Build history of the part. All positions in model axes, mm. Face numbers are marked on the shaded views. A direction names the side the tool comes from. Round coordinates to 2 decimals unless told otherwise and drop trailing zeros. Write each loop counter-clockwise with the first axis right and the second up, starting at its lowest first coordinate (ties: lowest second). Pieces come first, ordered by that corner, then holes.
Item 1: Wall check: probe 1 along Y at (x, z) = (11, 4); probe 2 along Y at (x, z) = (18, 10); probe 3 along Z at (x, y) = (1.5, -13). Give the ranges that are in metal, low to high.
Item 2: 3-axis set-ups, long thin cutter, end or side, ignore diameter. For the marked faces 4, 5, 6 and 7: which of +Z, -Z, +X, -X, +Y, -Y reach the whole face in a straight line?
Item 3: Band-saw the part on B-B, the plane x = 21.5. Write the cut outline in (y, z), then the cut area to 3 significant figures.
Item 4: Band-saw the part on A-A, the plane y = 25. Write the cut outline in (x, z).
Item 5: Drop flat-ended pins along their axis: pin 1 Ø3 at (x, y) = (17, -3) entering from -Z; pin 2 Ø5 at (y, z) = (-24, 3) entering from +X; pin 3 Ø2 at (x, z) = (21, 9.5) entering from +Y. Give the stop position or say it passes through.
Item 6: Band-saw the part on D-D, the plane x = -7.2. Count the separate pieces of the cut face and the enclosed holes in it, then the cut area to 3 significant figures.
Item 7: Mould opens along Z. For the marked faces 1, 2 and 3 say: +Z half, -Z half, draft (parallel to the pull), parting line (faces both ways), or undercut.
Item 8: Band-saw the part on C-C, the plane z = 10. Write the cut outline in (x, y), then the cut area to 3 significant figures.
```python
from build123d import *

# Parameters (mm, degrees)
CROQUIS1_W             = 99.2
CROQUIS1_H             = 47
BASE_DEPTH             = 17.6
CROQUIS2_W             = 30.4
CROQUIS2_H             = 14.4
PLATES_DEPTH           = 40.8
CROQUIS4_W             = 2
CROQUIS4_H             = 2.8
WINDOW_LATERAL_1_DEPTH = 40.8
CROQUIS5_R             = 2
WINDOW_LATERAL_2_DEPTH = 2
WINDOW_LATERAL_3_START = -2
WINDOW_LATERAL_3_DEPTH = 2
CROQUIS7_W             = 30.4
CROQUIS7_H             = 2.8
WINDOW_BEHIND_1_DEPTH  = 6.2
WINDOW_BEHIND_2_DEPTH  = 59.973892529
CROQUIS9_R             = 2
WINDOW_BEHIND_3_DEPTH  = 59.973892529
WINDOW_BOTTOM_DEPTH    = 59.973892529
ROTOR_JOIN_1_DEPTH     = 4
CROQUIS12_R            = 1.4
ROTOR_JOIN_2_DEPTH     = 10.2
ROTOR_LIMIT_1_DEPTH    = 16
ROTOR_LIMIT_2_DEPTH    = 16


with BuildPart() as part:
    # Croquis1 → BASE (new body)
    with BuildSketch(Plane(origin=(0, 0, 0), x_dir=(0, 1, 0), z_dir=(0, 0, 1))):
        with Locations((0, 4.1)):
            Rectangle(CROQUIS1_W, CROQUIS1_H)
    extrude(amount=BASE_DEPTH)

    # Croquis2 → PLATES (cut)
    with BuildSketch(Plane(origin=(-27.6, 0, 0), x_dir=(0, -1, 0), z_dir=(-1, 0, 0))):
        with Locations((-32.4, 8.8)):
            Rectangle(CROQUIS2_W, CROQUIS2_H)
        with Locations((0, 8.8)):
            Rectangle(CROQUIS2_W, CROQUIS2_H)
        with Locations((32.4, 8.8)):
            Rectangle(CROQUIS2_W, CROQUIS2_H)
    extrude(amount=-PLATES_DEPTH, mode=Mode.SUBTRACT)

    # Croquis4 → WINDOW_LATERAL_1 (cut)
    with BuildSketch(Plane(origin=(-27.6, 0, 0), x_dir=(0, -1, 0), z_dir=(-1, 0, 0))):
        with Locations((48.6, 14.6)):
            Rectangle(CROQUIS4_W, CROQUIS4_H)
        with Locations((-48.6, 14.6)):
            Rectangle(CROQUIS4_W, CROQUIS4_H)
    extrude(amount=-WINDOW_LATERAL_1_DEPTH, mode=Mode.SUBTRACT)

    # Croquis5 → WINDOW_LATERAL_2 (cut)
    with BuildSketch(Plane.XZ.offset(49.6)):
        with Locations((-7.2, 13.2)):
            Circle(CROQUIS5_R)
    extrude(amount=-WINDOW_LATERAL_2_DEPTH, mode=Mode.SUBTRACT)

    # Croquis6 → WINDOW_LATERAL_3 (cut)
    with BuildSketch(Plane(origin=(0, 49.6, 0), x_dir=(-1, 0, 0), z_dir=(0, 1, 0)).offset(WINDOW_LATERAL_3_START)):
        with BuildLine():
            Line((9.2, 13.2), (5.2, 13.2))
            ThreePointArc((5.2, 13.2), (7.2, 11.2), (9.2, 13.2))
        make_face()
    extrude(amount=WINDOW_LATERAL_3_DEPTH, mode=Mode.SUBTRACT)

    # Croquis7 → WINDOW_BEHIND_1 (cut)
    with BuildSketch(Plane(origin=(13.2, 0, 0), x_dir=(0, -1, 0), z_dir=(-1, 0, 0))):
        with Locations((0, 3)):
            Rectangle(CROQUIS7_W, CROQUIS7_H)
    extrude(amount=-WINDOW_BEHIND_1_DEPTH, mode=Mode.SUBTRACT)

    # Croquis8 → WINDOW_BEHIND_2 (cut, through all)
    with BuildSketch(Plane.XY.offset(1.6)):
        with BuildLine():
            Line((15.2, -11), (15.2, 11))
            ThreePointArc((15.2, 11), (19.4, 15.2), (23.6, 11))
            Line((23.6, 11), (23.6, -11))
            ThreePointArc((23.6, -11), (19.4, -15.2), (15.2, -11))
        make_face()
    extrude(amount=-WINDOW_BEHIND_2_DEPTH, mode=Mode.SUBTRACT)

    # Croquis9 → WINDOW_BEHIND_3 (cut, through all)
    with BuildSketch(Plane.XY.offset(1.6)):
        with Locations((15.2, 0)):
            Circle(CROQUIS9_R)
    extrude(amount=-WINDOW_BEHIND_3_DEPTH, mode=Mode.SUBTRACT)

    # Croquis10 → WINDOW_BOTTOM (cut, through all)
    with BuildSketch(Plane.XY.offset(1.6)):
        with BuildLine():
            Line((5.2, 11.2), (-19.6, 11.2))
            ThreePointArc((-19.6, 11.2), (-21.014213562, 10.614213562), (-21.6, 9.2))
            Line((-21.6, 9.2), (-21.6, -9.2))
            ThreePointArc((-21.6, -9.2), (-21.014213562, -10.614213562), (-19.6, -11.2))
            Line((-19.6, -11.2), (5.2, -11.2))
            ThreePointArc((5.2, -11.2), (6.614213562, -10.614213562), (7.2, -9.2))
            Line((7.2, -9.2), (7.2, 9.2))
            ThreePointArc((7.2, 9.2), (6.614213562, 10.614213562), (5.2, 11.2))
        make_face()
        with BuildLine():
            Line((7.2, 41.6), (7.2, 23.2))
            ThreePointArc((7.2, 23.2), (6.614213562, 21.785786438), (5.2, 21.2))
            Line((5.2, 21.2), (-19.6, 21.2))
            ThreePointArc((-19.6, 21.2), (-21.014213562, 21.785786438), (-21.6, 23.2))
            Line((-21.6, 23.2), (-21.6, 41.6))
            ThreePointArc((-21.6, 41.6), (-21.014213562, 43.014213562), (-19.6, 43.6))
            Line((-19.6, 43.6), (5.2, 43.6))
            ThreePointArc((5.2, 43.6), (6.614213562, 43.014213562), (7.2, 41.6))
        make_face()
        with BuildLine():
            Line((5.2, -21.2), (-19.6, -21.2))
            ThreePointArc((-19.6, -21.2), (-21.014213562, -21.785786438), (-21.6, -23.2))
            Line((-21.6, -23.2), (-21.6, -41.6))
            ThreePointArc((-21.6, -41.6), (-21.014213562, -43.014213562), (-19.6, -43.6))
            Line((-19.6, -43.6), (5.2, -43.6))
            ThreePointArc((5.2, -43.6), (6.614213562, -43.014213562), (7.2, -41.6))
            Line((7.2, -41.6), (7.2, -23.2))
            ThreePointArc((7.2, -23.2), (6.614213562, -21.785786438), (5.2, -21.2))
        make_face()
    extrude(amount=-WINDOW_BOTTOM_DEPTH, mode=Mode.SUBTRACT)

    # Croquis11 → ROTOR_JOIN_1 (add)
    with BuildSketch(Plane.YZ.offset(19.4)):
        with BuildLine():
            Line((-10, 14), (10, 14))
            ThreePointArc((10, 14), (11.414213562, 13.414213562), (12, 12))
            Line((12, 12), (12, 8))
            ThreePointArc((12, 8), (11.414213562, 6.585786438), (10, 6))
            Line((10, 6), (-10, 6))
            ThreePointArc((-10, 6), (-11.414213562, 6.585786438), (-12, 8))
            Line((-12, 8), (-12, 12))
            ThreePointArc((-12, 12), (-11.414213562, 13.414213562), (-10, 14))
        make_face()
    extrude(amount=ROTOR_JOIN_1_DEPTH)

    # Croquis12 → ROTOR_JOIN_2 (cut)
    with BuildSketch(Plane.YZ.offset(23.4)):
        with Locations(Location((0, 10, 0), (0, 0, 270))):
            Circle(CROQUIS12_R)
    extrude(amount=-ROTOR_JOIN_2_DEPTH, mode=Mode.SUBTRACT)

    # Croquis14 → ROTOR_LIMIT_1 (add)
    with BuildSketch(Plane.XZ.offset(49.6)):
        Polygon((19.4, 0), (19.4, 3.2), (25, 0), align=None)
    extrude(amount=-ROTOR_LIMIT_1_DEPTH)

    # Croquis15 → ROTOR_LIMIT_2 (add)
    with BuildSketch(Plane(origin=(0, 49.6, 0), x_dir=(-1, 0, 0), z_dir=(0, 1, 0))):
        Polygon((-25, 0), (-19.4, 0), (-19.4, 3.2), align=None)
    extrude(amount=-ROTOR_LIMIT_2_DEPTH)


solid = part.part
```
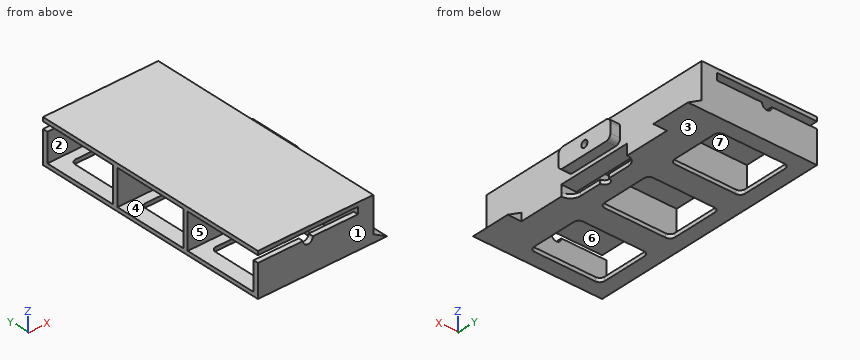
Results:
1. probe 1: y = -49.6 to -47.6, -17.2 to -15.2, 15.2 to 17.2, 47.6 to 49.6
1. probe 2: y = -49.6 to -1.4, 1.4 to 49.6
1. probe 3: z = 0 to 1.6, 16 to 17.6
2. face 4: +X, -X
2. face 5: -X
2. face 6: -X, -Y
2. face 7: -X, +Y
3. outline: (-49.6, 0) - (-33.6, 0) - (-33.6, 2) - (-49.6, 2) - close; (-12, 8) arc R2 ccw to (-10, 6) - (10, 6) arc R2 ccw to (12, 8) - (12, 12) arc R2 ccw to (10, 14) - (-10, 14) arc R2 ccw to (-12, 12) - close; (33.6, 0) - (49.6, 0) - (49.6, 2) - (33.6, 2) - close; hole circle Ø2.8 at (0, 10)
3. area: 246 mm2
4. outline: (-27.6, 0) - (-21.6, 0) - (-21.6, 1.6) - (-27.6, 1.6) - close; (-27.6, 16) - (13.2, 16) - (13.2, 1.6) - (7.2, 1.6) - (7.2, 0) - (19.4, 0) - (19.4, 17.6) - (-27.6, 17.6) - close
5. pin 1: stops at z = 4.4
5. pin 2: stops at x = 19.4
5. pin 3: stops at y = 12
6. separate pieces: 3
6. enclosed holes: 0
6. area: 306 mm2
7. face 1: draft
7. face 2: undercut
7. face 3: -Z half
8. outline: (-27.6, -49.6) - (19.4, -49.6) - (19.4, -12) - (23.4, -12) - (23.4, -1.4) - (13.2, -1.4) - (13.2, -15.2) - (-27.6, -15.2) - (-27.6, -17.2) - (13.2, -17.2) - (13.2, -47.6) - (-27.6, -47.6) - close; (-27.6, 15.2) - (13.2, 15.2) - (13.2, 1.4) - (23.4, 1.4) - (23.4, 12) - (19.4, 12) - (19.4, 49.6) - (-27.6, 49.6) - (-27.6, 47.6) - (13.2, 47.6) - (13.2, 17.2) - (-27.6, 17.2) - close
8. area: 1,010 mm2
